from build123d import *

# Parameters (mm, degrees)
MAIN_DEPTH        = 30
FIX_2_DEPTH       = 1
SKETCH4_R         = 1.6
FIXHOLE_DEPTH     = 32
SKETCH6_R         = 4.25
FIXTOOLHOLE_DEPTH = 10


with BuildPart() as part:
    # Sketch1 → Main (new body)
    with BuildSketch(Plane.XY):
        with BuildLine():
            Line((4.012678164, 8.096844755), (4.012678164, 9.096844755))
            ThreePointArc((4.012678164, 9.096844755), (10.635131042, 14.159397508), (16.012678164, 20.528723174))
            Line((16.012678164, 20.528723174), (20.012678164, 20.528723174))
            ThreePointArc((20.012678164, 20.528723174), (25.237773803, 13.999369756), (32.012678164, 9.096844755))
            Line((32.012678164, 9.096844755), (32.012678164, 8.096844755))
            Line((32.012678164, 8.096844755), (4.012678164, 8.096844755))
        make_face()
    extrude(amount=MAIN_DEPTH)

    # Sketch5 → Fix 2 (add)
    with BuildSketch(Plane.XY.offset(30)):
        with BuildLine():
            Line((11.035981199, 14.546844755), (24.677385704, 14.546844755))
            ThreePointArc((24.677385704, 14.546844755), (26.295048181, 13.037479939), (28.015846782, 11.646844755))
            Line((28.015846782, 11.646844755), (7.71870745, 11.646844755))
            ThreePointArc((7.71870745, 11.646844755), (9.418864977, 13.0493498), (11.035981199, 14.546844755))
        make_face()
    extrude(amount=FIX_2_DEPTH)

    # Sketch4 → FixHole (cut, through all)
    with BuildSketch(Plane.XY.offset(31)):
        with Locations((18.012678164, 13.096844755)):
            Circle(SKETCH4_R)
    extrude(amount=-FIXHOLE_DEPTH, mode=Mode.SUBTRACT)

    # Sketch6 → FixToolHole (cut)
    with BuildSketch(Plane(origin=(0, 0, 0), x_dir=(-1, 0, 0), z_dir=(0, 0, -1))):
        with Locations((-18.012678164, 13.096844755)):
            Circle(SKETCH6_R)
    extrude(amount=-FIXTOOLHOLE_DEPTH, mode=Mode.SUBTRACT)


solid = part.part
Read the model definition and answer for the solid it produces. Units are mm, in the model's axes. A direction names the side the tool comes from. Coordinates: 2 decimals unless noted, no trailing zeros. Write each loop counter-clockwise with the first axis right and the second up, starting at its lowest first coordinate (ties: lowest second). Pieces come first, ordered by that corner, then holes. Notation, with made-up numbers: (38.5, -33.75) - (95.5, -33.75) arc R19 ccw to (95.5, -6.75) - close; hole circle Ø3 at (-22, 58.5). An arc over 180 degrees is marked (long way). One line per question, with ' | ' between items.
Q1. Find section B-B, the plane x = 9.25. Write down the section's boundary in (y, z), plus the area to 3 significant figures.
Result set:
outline: (8.1, 0) - (12.9, 0) - (12.9, 31) - (11.65, 31) - (11.65, 30) - (8.1, 30) - close | area: 145 mm^2
Q2. Find section A-A, the plane z = 26. Write down the section's boundary in (x, y).
Result set:
outline: (4.01, 8.1) - (32.01, 8.1) - (32.01, 9.1) arc R31.12 cw to (20.01, 20.53) - (16.01, 20.53) arc R38.5 cw to (4.01, 9.1) - close; hole circle Ø3.2 at (18.01, 13.1)
Q3. Determine the mould class of faces 1 (the flat face through (14.1, 14.547, 30.5)), 2 (the flat face through (13, 13, 31)), 3 (the flat face through (18, 11, 10)) for opening direction Y: +Y half, -Y half, draft (parallel to the pull), parting line (faces both ways), or undercut.
Result set:
face 1: +Y half | face 2: draft | face 3: undercut
Q4. Find section D-D, the plane z = 5.5. Write down the section's boundary in (x, y), plus the area to 3 significant figures.
Result set:
outline: (4.01, 8.1) - (32.01, 8.1) - (32.01, 9.1) arc R31.12 cw to (20.01, 20.53) - (16.01, 20.53) arc R38.5 cw to (4.01, 9.1) - close; hole circle Ø8.5 at (18.01, 13.1) | area: 132 mm^2
Q5. Each of these flat-tipped pins is pushed along its axis until it touches: P1, Ø1.1, axis at x = 12, y = 10, coming from the +Z side; P2, Ø6.5, axis at x = 18, y = 16.5, coming from the +Z side; P3, Ø1, axis at y = 17.5, z = 17.5, coming from the -X side; P4, Ø2, axis at y = 13.5, z = 13, coming from the -X side. Where does it stop, or does it pass through?
Result set:
P1: z = 30 | P2: z = 31 | P3: x = 13.33 | P4: x = 8.78
Q6. For faces 4 (the flat face through (12.6, 11.647, 30.5)), 5 (the flat face through (18, 17, 30)), 6 (the cylindrical face through (21.385, 10.511, 4.93)), determine the directions among +Z, -Z, +X, -X, +Y, -Y from which every point of the face is accessible in a straight line to the end or side of a thin tool.
Result set:
face 4: +Z, +X, -X, -Y | face 5: +Z, +X, -X, +Y | face 6: -Z
Q7. Consider L1, parallel to Y at x = 18, z = 10.5; L2, parallel to X at y = 14.5, z = 7; L3, parallel to Z at x = 14.25, y = 16. Determine where each line is inside the solid, lowest interval first. Write a range as [from, to].
Result set:
L1: [8.1, 11.5], [14.7, 20.53] | L2: [10.99, 14], [22.02, 24.72] | L3: [0, 30]
Q8. Find section C-C, the plane y = 16. Write down the section's boundary in (x, z).
Result set:
outline: (12.44, 0) - (14.91, 0) - (14.91, 10) - (21.12, 10) - (21.12, 0) - (23.32, 0) - (23.32, 30) - (12.44, 30) - close
